```python
from build123d import *

# Parameters (mm, degrees)
F0_W      = 35
F0_H      = 250
F1_DEPTH  = 45
F3_DEPTH  = 250
F4_DEPTH  = 250
F5_R      = 8.5849434278
F6_T      = -2.54
F7_W      = 6.1992760748
F7_H      = 72.0517709851
F8_DEPTH  = 80
F10_DEPTH = 101.346


# Not quite as in the source:
# - a shell that OpenCascade refuses in one call is made with other operations: the cavity is built on its own and cut out
# - a feature names something its author has since deleted; it is built from what else it names


with BuildPart() as f1:
    # F0 (on Top) → F1 (new body)
    with BuildSketch(Plane.XY):
        with Locations((17.5, -125)):
            Rectangle(F0_W, F0_H)
    extrude(amount=-F1_DEPTH)

    # F2 (on face) → F3 (join)
    with BuildSketch(Plane(origin=(0, 0, 0), x_dir=(-1, 0, 0), z_dir=(0, 1, 0))):
        with BuildLine():
            Line((-17.5, -45), (0, -45))
            ThreePointArc((0, -45), (-5.1256313292, -32.6256313292), (-17.5, -27.5))
            ThreePointArc((-17.5, -27.5), (-29.8743686708, -32.6256313292), (-35, -45))
            Line((-35, -45), (-17.5, -45))
        make_face()
        with BuildLine():
            ThreePointArc((-35, -45), (-17.5, -62.5), (0, -45))
            Line((0, -45), (-17.5, -45))
            Line((-17.5, -45), (-35, -45))
        make_face()
        with BuildLine():
            ThreePointArc((-17.5, -27.5), (-5.1256313292, -32.6256313292), (0, -45))
            Line((0, -45), (0, -27.5))
            Line((0, -27.5), (-17.5, -27.5))
        make_face()
    extrude(amount=-F3_DEPTH)

    # F2 (on face) → F4 (join)
    with BuildSketch(Plane(origin=(0, 0, 0), x_dir=(-1, 0, 0), z_dir=(0, 1, 0))):
        with BuildLine():
            Line((-17.5, -45), (0, -45))
            ThreePointArc((0, -45), (-5.1256313292, -32.6256313292), (-17.5, -27.5))
            ThreePointArc((-17.5, -27.5), (-29.8743686708, -32.6256313292), (-35, -45))
            Line((-35, -45), (-17.5, -45))
        make_face()
        with BuildLine():
            ThreePointArc((-35, -45), (-17.5, -62.5), (0, -45))
            Line((0, -45), (-17.5, -45))
            Line((-17.5, -45), (-35, -45))
        make_face()
        with BuildLine():
            ThreePointArc((-17.5, -27.5), (-5.1256313292, -32.6256313292), (0, -45))
            Line((0, -45), (0, -27.5))
            Line((0, -27.5), (-17.5, -27.5))
        make_face()
    extrude(amount=-F4_DEPTH)

    # F5
    f5_edges = [f1.edges().sort_by_distance(p)[0] for p in [
        (17.5, 0, 0),
        (35, 0, -22.5),
        (17.5, 0, -62.5),
        (0, 0, -22.5),
        (17.5, -250, 0),
        (0, -250, -22.5),
        (17.5, -250, -62.5),
        (35, -250, -22.5),
    ]]
    fillet(f5_edges, radius=F5_R)

    # F6: a shell. OpenCascade refuses it in one call, so the cavity is built on its own and cut out:
    # the body offset inwards by the wall thickness, plus a prism from it out through each open face.
    f6_core = offset(f1.part, amount=F6_T, mode=Mode.PRIVATE)
    f6_exits = [f6_core.faces().sort_by_distance(p)[0] for p in [
        (17.5, -125, -2.54),
    ]]
    add(f6_core, mode=Mode.SUBTRACT)
    extrude(f6_exits, amount=-F6_T, mode=Mode.SUBTRACT)

    # F7 (on Top) → F8 (join)
    with BuildSketch(Plane.XY):
        with Locations((17.7442375571, -36.0258854926)):
            Rectangle(F7_W, F7_H)
    extrude(amount=-F8_DEPTH)

    # F9 (on face) → F10 (cut)
    with BuildSketch(Plane.XZ.offset(72.0517709851)):
        Polygon((16.4569599832, -69.1932439804), (16.4569599832, -62.46888856), (14.6445995197, -62.5368878245), (14.6445995197, -69.1932439804), align=None)
        Polygon((20.8438755944, -62.1775579175), (19.5716265936, -62.376949193), (19.5716265936, -69.1005588385), (20.8438755944, -69.1005588385), align=None)
    extrude(amount=-F10_DEPTH, mode=Mode.SUBTRACT)


solid = f1.part
```
Could you check a few things on this model? Use its own coordinates, in mm. A direction names the side the tool comes from. Coordinates: 2 decimals unless noted, no trailing zeros. Write each loop counter-clockwise with the first axis right and the second up, starting at its lowest first coordinate (ties: lowest second). Pieces come first, ordered by that corner, then holes. Notation, with made-up numbers: M -26.75,-21 L 13.25,-21 A17 ccw 13.25,-6 Z; hole C 72.25,84 d10. An arc over 180 degrees is marked long. Answer as CSV lines item,"result". Start each with the question number.
1) I want a section at A-A, the plane z = -12. Please give me the cut outline in (x, y), and give its area (3 significant figures).
2) For P1, Ø5, axis at y = -47, z = -71.5, coming from the -X side; P2, Ø5, axis at x = 17.5, z = -67.5, coming from the -Y side; P3, Ø10, axis at y = -180.5, z = -66, coming from the -X side, each with a flat end and sliding along its axis, tell me the tip position at first contact or that it passes through.
3) I want a section at C-C, the plane y = -63.5. Please give me the cut outline in (x, z).
4) Please list where these lines run through material, in increasing order: line 1 (X direction, y = -22.5, z = -18.5); line 2 (X direction, y = -158.5, z = -18); line 3 (Y direction, x = 15, z = -19). Write a range as from..to.
5) I want a section at B-B, the plane y = -114. Please give me the cut outline in (x, z).
6) For faces 1 (the flat face through (14.645, -2, -2)), 2 (the flat face through (19.572, -37, -66)), 3 (the flat face through (18, -72.052, -30)), 4 (the cylindrical face through (25.44, -4.36, -4.26)), which set-ups out of +Z, -Z, +X, -X, +Y, -Y let a thin tool reach every point of the face, with its end or its side?
7) We'd pull the mould along Z, two halves only. Please class faces 5 (the cylindrical face through (26.45, -3.74, -1.5)), 6 (the flat face through (18, -72.052, -73)), 7 (the cylindrical face through (30.64, -4.26, -24.07)): +Z half, -Z half, draft (parallel to the pull), parting line (faces both ways), or undercut.
Data:
1,outline,"M 0,-241.42 A8.58 ccw 8.58,-250 L 26.42,-250 A8.58 ccw 35,-241.42 L 35,-8.58 A8.58 ccw 26.42,0 L 8.58,0 A8.58 ccw 0,-8.58 Z; hole M 2.54,-241.42 A6.04 ccw 8.58,-247.46 L 26.42,-247.46 A6.04 ccw 32.46,-241.42 L 32.46,-8.58 A6.04 ccw 26.42,-2.54 L 20.84,-2.54 L 20.84,-72.05 L 14.64,-72.05 L 14.64,-2.54 L 8.58,-2.54 A6.04 ccw 2.54,-8.58 Z"
1,area,"1,820 mm^2"
2,P1,"stops at x = 14.64"
2,P2,"stops at y = -72.05"
2,P3,"stops at x = 10.41"
3,outline,"M 0,-45 A17.5 ccw 14.64,-62.27 L 14.64,-62.54 L 16.46,-62.47 L 16.46,-69.19 L 14.64,-69.19 L 14.64,-80 L 20.84,-80 L 20.84,-69.1 L 19.57,-69.1 L 19.57,-62.38 L 20.84,-62.18 A17.5 ccw 35,-45 L 35,0 L 32.46,0 L 32.46,-45 A14.96 cw 20.84,-59.58 L 20.84,0 L 14.64,0 L 14.64,-59.68 A14.96 cw 2.54,-45 L 2.54,0 L 0,0 Z"
4,line 1,"x = 0..2.54, 14.64..20.84, 32.46..35"
4,line 2,"x = 0..2.54, 32.46..35"
4,line 3,"y = -250..-247.46, -72.05..0"
5,outline,"M 0,-45 A17.5 ccw 35,-45 L 35,0 L 32.46,0 L 32.46,-45 A14.96 cw 2.54,-45 L 2.54,0 L 0,0 Z"
6,face 1,"+Z, -X, +Y"
6,face 2,"+X, +Y, -Y"
6,face 3,"+Z"
6,face 4,"none"
7,face 5,"+Z half"
7,face 6,"draft"
7,face 7,"undercut"
